Verification items for the finished model (mm, model axes). A direction names the side the tool comes from. Coordinates: 2 decimals unless noted, no trailing zeros. Order: outer loops, then holes, each group sorted by start corner. A loop starts at its lowest first (then second) coordinate and runs counter-clockwise, first axis right, second up. Notation, with made-up numbers: (48.25, 58.25) -> (107.25, 58.25) arc R17 cw to (107.25, 82.25) -> close; hole circle Ø7 at (9.5, 41). An arc over 180 degrees is marked (long way). Write each question's results on one line, items separated by ' | '. Start each with the question number.
(1) Cross-section at B-B on y = -1.5. Enter the section's corners in (x, z), and give its area (3 significant figures).
(2) Go/stop test with flat-tipped pins: pin 1 (2 mm diameter, centred on x = 0, z = 5, fed in from -Y); pin 2 (1.2 mm diameter, centred on y = 6.5, z = 10, fed in from +X); pin 3 (6.5 mm diameter, centred on x = 0, z = 5, fed in from -Y) (3 decimals). Record where each tip stops, or that it passes through.
(3) Thickness scan on probe 1 along X at (y, z) = (-15, 3.5); probe 2 along X at (y, z) = (5, 6.25); probe 3 along X at (y, z) = (-12.5, 11.5). Record the ranges inside material, lowest first. Write a range as [from, to].
(4) Draft check along Y on faces 4 (the cylindrical face through (-23.61, -16.67, 7.4)), 5 (the flat face through (9, -10.375, 7)), 6 (the cylindrical face through (-13.97, -8.1, 7.4)), 7 (the cylindrical face through (-26.156, -10.524, 7.395)). Enter one of: +Y half, -Y half, draft (parallel to the pull), parting line (faces both ways), or undercut.
(5) Cross-section at A-A on x = -8. Enter the section's corners in (y, z) (3 decimals), and give its area (3 significant figures).
(6) Set-up check for faces 1 (the cylindrical face through (13.92, 7.5, 8.57)), 2 (the cylindrical face through (21.23, -6.82, 3.06)), 3 (the cylindrical face through (14, -8.05, 7.4)): record each of +Z, -Z, +X, -X, +Y, -Y from which the full face is reachable in a straight line by a thin tool's end or side.
(7) Cross-section at C-C on z = 5. Give the number of separate pieces and of enclosed holes in the cut face, and give its area (3 significant figures).
(8) Cross-section at D-D on x = 0. Enter the section's corners in (y, z) (3 decimals).
```python
from build123d import *

# Parameters (mm, degrees)
SKETCH_1_R               = 2.6
EXTRUDE_1_DEPTH          = 15
CUT_EXTRUDE_1_REACH      = 58.014
CUT_EXTRUDE_1_END_RADIUS = 6
SKETCH_3_R               = 2
SKETCH_4_R               = 3.6
CUT_EXTRUDE_2_DEPTH      = 4.2
SKETCH_6_R               = 5.1
CUT_EXTRUDE_4_DEPTH      = 6.2
CUT_EXTRUDE_5_REACH      = 53.779
CUT_EXTRUDE_5_END_RADIUS = 6
SKETCH_7_R               = 2
SKETCH_8_R               = 3.6
CUT_EXTRUDE_6_DEPTH      = 4.2
CUT_EXTRUDE_7_DEPTH      = 43.095434039
FILLET_1_R               = 0.5


with BuildPart() as part:
    # ｽｹｯﾁ1 → ﾎﾞｽ - 押し出し1 (new body)
    with BuildSketch(Plane.XY):
        with BuildLine():
            ThreePointArc((1.060449829, 29.107252287), (-2.678502383, 28.760723475), (-5.479274058, 26.259618943))
            Line((-5.479274058, 26.259618943), (-25.394531587, -8.234618943))
            ThreePointArc((-25.394531587, -8.234618943), (-26.160165812, -10.558527256), (-25.934363924, -12.994868595))
            Line((-25.934363924, -12.994868595), (-25.737844829, -13.635249652))
            ThreePointArc((-25.737844829, -13.635249652), (-23.56826597, -16.700012845), (-20.00186007, -17.875))
            Line((-20.00186007, -17.875), (19.828654989, -17.875))
            ThreePointArc((19.828654989, -17.875), (22.224035736, -17.376104532), (24.221068284, -15.962383691))
            Line((24.221068284, -15.962383691), (24.677395, -15.472002635))
            ThreePointArc((24.677395, -15.472002635), (26.246768352, -12.06071063), (25.481134127, -8.384618943))
            Line((25.481134127, -8.384618943), (5.565876598, 26.109618943))
            ThreePointArc((5.565876598, 26.109618943), (3.936130075, 27.934631788), (1.713295639, 28.957252287))
            Line((1.713295639, 28.957252287), (1.060449829, 29.107252287))
        make_face()
        with Locations((-20.56810334, -11.875)):
            Circle(SKETCH_1_R, mode=Mode.SUBTRACT)
        with BuildLine():
            ThreePointArc((6, 0), (-3.464101615, -4.898979486), (-2, 5.656854249))
            Line((-2, 5.656854249), (-2, 8))
            Line((-2, 8), (2, 8))
            Line((2, 8), (2, 5.656854249))
            ThreePointArc((2, 5.656854249), (4.898979486, 3.464101615), (6, 0))
        make_face(mode=Mode.SUBTRACT)
        with Locations((20.56810334, -11.875)):
            Circle(SKETCH_1_R, mode=Mode.SUBTRACT)
        with Locations((0, 23.75)):
            Circle(SKETCH_1_R, mode=Mode.SUBTRACT)
    extrude(amount=EXTRUDE_1_DEPTH)

    # ｶｯﾄ - 押し出し1: up to this cylinder (the profile starts outside it)
    cut_extrude_1_end = Plane(origin=(0, 0, 5), z_dir=(0, 0, -1)) * Cylinder(CUT_EXTRUDE_1_END_RADIUS, 129.028, mode=Mode.PRIVATE)
    # ｽｹｯﾁ3 → ｶｯﾄ - 押し出し1 (cut, up to the surface)
    with BuildSketch(Plane.XZ.offset(17.875), mode=Mode.PRIVATE) as cut_extrude_1_sk1:
        with Locations(Location((0, 5, 0), (0, 0, 270))):
            Circle(SKETCH_3_R)
    cut_extrude_1_tool1 = extrude(cut_extrude_1_sk1.sketch, amount=-CUT_EXTRUDE_1_REACH, mode=Mode.PRIVATE) - cut_extrude_1_end
    add(cut_extrude_1_tool1.solids().sort_by_distance((0, -17.875, 5))[0], mode=Mode.SUBTRACT)

    # ｽｹｯﾁ4 → ｶｯﾄ - 押し出し2 (cut)
    with BuildSketch(Plane.XZ.offset(17.875)):
        with Locations(Location((0, 5, 0), (0, 0, 270))):
            Circle(SKETCH_4_R)
    extrude(amount=-CUT_EXTRUDE_2_DEPTH, mode=Mode.SUBTRACT)

    # ｽｹｯﾁ6 → ｶｯﾄ - 押し出し4 (cut)
    with BuildSketch(Plane(origin=(0, 0, 0), x_dir=(-1, 0, 0), z_dir=(0, 0, -1))):
        with Locations((0, 23.75)):
            Circle(SKETCH_6_R)
        with Locations((-20.56810334, -11.875)):
            Circle(SKETCH_6_R)
        with Locations((20.56810334, -11.875)):
            Circle(SKETCH_6_R)
    extrude(amount=-CUT_EXTRUDE_4_DEPTH, mode=Mode.SUBTRACT)

    # ｶｯﾄ - 押し出し5: up to this cylinder (the profile starts outside it)
    cut_extrude_5_end = Plane(origin=(0, 0, 5), z_dir=(0, 0, -1)) * Cylinder(CUT_EXTRUDE_5_END_RADIUS, 120.558, mode=Mode.PRIVATE)
    # ｽｹｯﾁ7 → ｶｯﾄ - 押し出し5 (cut, up to the surface)
    with BuildSketch(Plane(origin=(15.480204093, 8.9375, 0), x_dir=(0, 0, -1), z_dir=(0.8660254037844386, 0.5000000000000001, 0)), mode=Mode.PRIVATE) as cut_extrude_5_sk1:
        with Locations(Location((-5, 0, 0), (0, 0, 90))):
            Circle(SKETCH_7_R)
    cut_extrude_5_tool1 = extrude(cut_extrude_5_sk1.sketch, amount=-CUT_EXTRUDE_5_REACH, mode=Mode.PRIVATE) - cut_extrude_5_end
    add(cut_extrude_5_tool1.solids().sort_by_distance((15.480204, 8.9375, 5))[0], mode=Mode.SUBTRACT)

    # ｽｹｯﾁ8 → ｶｯﾄ - 押し出し6 (cut)
    with BuildSketch(Plane(origin=(15.480204093, 8.9375, 0), x_dir=(0, 0, -1), z_dir=(0.8660254037844386, 0.5000000000000001, 0))):
        with Locations(Location((-5, 0, 0), (0, 0, 90))):
            Circle(SKETCH_8_R)
    extrude(amount=-CUT_EXTRUDE_6_DEPTH, mode=Mode.SUBTRACT)

    # ｽｹｯﾁ9 → ｶｯﾄ - 押し出し7 (cut, through all)
    with BuildSketch(Plane(origin=(0, 0, 0), x_dir=(-1, 0, 0), z_dir=(0, 0, -1))):
        with BuildLine():
            ThreePointArc((2.426213564, 16.547674838), (0, 16.15), (-2.426213564, 16.547674838))
            Line((-2.426213564, 16.547674838), (-7.157489625, 8.352864316))
            ThreePointArc((-7.157489625, 8.352864316), (0, 11), (7.157489625, 8.352864316))
            Line((7.157489625, 8.352864316), (2.426213564, 16.547674838))
        make_face()
        with BuildLine():
            ThreePointArc((-3.655047879, -10.375), (-9.526279442, -5.5), (-10.812537504, 2.022135684))
            Line((-10.812537504, 2.022135684), (-15.543813565, -6.172674838))
            ThreePointArc((-15.543813565, -6.172674838), (-13.986310271, -8.075), (-13.117600001, -10.375))
            Line((-13.117600001, -10.375), (-3.655047879, -10.375))
        make_face()
        with BuildLine():
            Line((15.543813565, -6.172674838), (10.812537504, 2.022135684))
            ThreePointArc((10.812537504, 2.022135684), (9.526279442, -5.5), (3.655047879, -10.375))
            Line((3.655047879, -10.375), (13.117600001, -10.375))
            ThreePointArc((13.117600001, -10.375), (13.986310271, -8.075), (15.543813565, -6.172674838))
        make_face()
    extrude(amount=-CUT_EXTRUDE_7_DEPTH, mode=Mode.SUBTRACT)

    # ﾌｨﾚｯﾄ1
    fillet_1_edges = [part.edges().sort_by_distance(p)[0] for p in [
        (13.117600001, -10.375, 7.5),
        (15.543813565, -6.172674838, 7.5),
        (10.812537504, 2.022135684, 7.5),
        (3.655047879, -10.375, 7.5),
        (2.426213564, 16.547674838, 7.5),
        (-2.426213564, 16.547674838, 7.5),
        (-7.157489625, 8.352864316, 7.5),
        (7.157489625, 8.352864316, 7.5),
        (-15.543813565, -6.172674838, 7.5),
        (-13.117600001, -10.375, 7.5),
        (-3.655047879, -10.375, 7.5),
        (-10.812537504, 2.022135684, 7.5),
    ]]
    fillet(fillet_1_edges, radius=FILLET_1_R)


solid = part.part
```
Results are:
1) outline: (-21.51, 0) -> (-12.85, 0) -> (-12.85, 15) -> (-21.51, 15) -> close; (-10.9, 0) -> (-5.81, 0) -> (-5.81, 15) -> (-10.9, 15) -> close; (5.81, 0) -> (10.9, 0) -> (10.9, 15) -> (5.81, 15) -> close; (12.85, 0) -> (21.51, 0) -> (21.51, 15) -> (12.85, 15) -> close | area: 412 mm2
2) pin 1: stops at y = 8 | pin 2: stops at x = 17.23 | pin 3: stops at y = -13.675
3) probe 1: x = [-25.12, -24.6], [-16.54, -3.27], [3.27, 16.54], [24.6, 25.07] | probe 2: x = [-17.75, -3.32], [3.32, 5.54], [11.78, 12.9], [15.41, 17.75] | probe 3: x = [-26.06, -23.09], [-18.04, 18.04], [23.09, 26.18]
4) face 4: -Y half | face 5: undercut | face 6: undercut | face 7: parting line
5) outline: (-17.875, 0) -> (-10.375, 0) -> (-10.375, 15) -> (-17.875, 15) -> close; (-7.55, 0) -> (21.894, 0) -> (21.894, 15) -> (-7.55, 15) -> close | area: 554 mm2
6) face 1: none | face 2: -Z | face 3: +Z, -Z
7) separate pieces: 2 | enclosed holes: 6 | area: 935 mm2
8) outline: (-17.875, 0) -> (-6, 0) -> (-6, 3) -> (-13.675, 3) -> (-13.675, 1.4) -> (-17.875, 1.4) -> close; (-17.875, 8.6) -> (-13.675, 8.6) -> (-13.675, 7) -> (-6, 7) -> (-6, 15) -> (-17.875, 15) -> close; (8, 0) -> (11, 0) -> (11, 15) -> (8, 15) -> close; (16.15, 0) -> (18.65, 0) -> (18.65, 6.2) -> (21.15, 6.2) -> (21.15, 15) -> (16.15, 15) -> close; (26.35, 6.2) -> (28.85, 6.2) -> (28.85, 0) -> (29.253, 0) -> (29.253, 15) -> (26.35, 15) -> close
